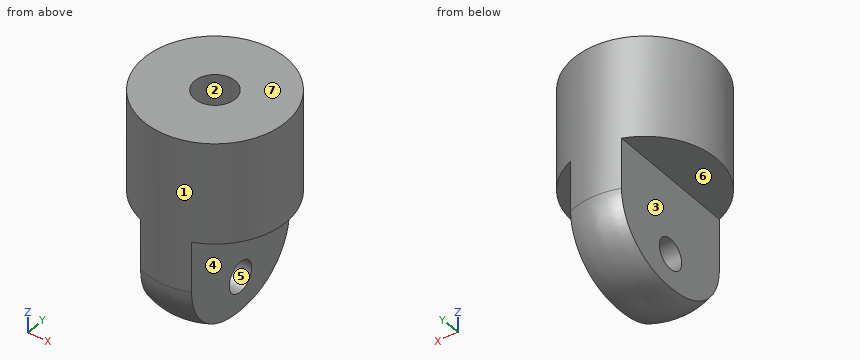
```python
from build123d import *

# Parameters (mm, degrees)
SKETCH2_R          = 4
CUT_EXTRUDE1_DEPTH = 30
SKETCH3_W          = 19.126095086
SKETCH3_H          = 32.253484506
SKETCH3_W_2        = 14.725893552
SKETCH3_H_2        = 25.816213186
CUT_EXTRUDE2_DEPTH = 15
SKETCH4_R          = 3
CUT_EXTRUDE3_DEPTH = 30


with BuildPart() as part:
    # Sketch1 → Revolve1 (revolve)
    with BuildSketch(Plane(origin=(0, 0, 0), x_dir=(0, 0, -1), z_dir=(1, 0, 0)), mode=Mode.PRIVATE) as revolve1_sk:
        with BuildLine():
            Line((0, 0), (0, 14))
            Line((0, 14), (30, 14))
            ThreePointArc((30, 14), (39.186081867, 9.751268794), (41.896907171, 0))
            Line((41.896907171, 0), (0, 0))
        make_face()
    revolve(revolve1_sk.sketch.rotate(Axis((0, 0, 8.753832377), (0, 0, -1)), 90), axis=Axis((0, 0, 8.753832377), (0, 0, -1)))

    # Sketch2 → Cut-Extrude1 (cut)
    with BuildSketch(Plane.XY):
        Circle(SKETCH2_R)
    extrude(amount=-CUT_EXTRUDE1_DEPTH, mode=Mode.SUBTRACT)

    # Sketch3 → Cut-Extrude2 (cut, symmetric)
    with BuildSketch(Plane(origin=(0, 0, 0), x_dir=(1, 0, 0), z_dir=(0, 1, 0))):
        with Locations((-14.563047543, 36.126742253)):
            Rectangle(SKETCH3_W, SKETCH3_H)
        with Locations((12.362946776, 32.908106593)):
            Rectangle(SKETCH3_W_2, SKETCH3_H_2)
    extrude(amount=CUT_EXTRUDE2_DEPTH, both=True, mode=Mode.SUBTRACT)

    # Sketch4 → Cut-Extrude3 (cut)
    with BuildSketch(Plane(origin=(5, 0, 0), x_dir=(0, 0, -1), z_dir=(1, 0, 0))):
        with Locations((35, 0)):
            Circle(SKETCH4_R)
    extrude(amount=-CUT_EXTRUDE3_DEPTH, mode=Mode.SUBTRACT)


solid = part.part
```
Geometry check sheet. Reference: the model listing, model coordinates, mm. Face numbers are marked on the shaded views. A direction names the side the tool comes from. Round coordinates to 2 decimals unless told otherwise and drop trailing zeros. Order: outer loops, then holes, each group sorted by start corner. A loop starts at its lowest first (then second) coordinate and runs counter-clockwise, first axis right, second up. Notation, with made-up numbers: M 26.5,59.25 L 35.5,59.25 A14 ccw 35.5,85.25 Z; hole C -5,57.5 d8. An arc over 180 degrees is marked long. Write item = value, one per line.
Q1. Depth check by flat-ended pin: pin 1 Ø7 at (x, y) = (-10, 1.5) entering from -Z; pin 2 Ø6.5 at (y, z) = (-5.5, -32.5) entering from +X; pin 3 Ø3.5 at (y, z) = (0, -35) entering from -X; pin 4 Ø6 at (x, y) = (-4.5, -8) entering from -Z. Enter the tip coordinate at first touch or a pass-through.
Answer block:
pin_1 = -20
pin_2 = 5
pin_3 = through
pin_4 = -41.29
Q2. Release check for a two-part mould opening along Z. For the marked faces 4, 5, 6 and 7 record: released by +Z, released by -Z, zero draft, split by the parting line, or undercut.
Answer block:
face_4 = zero draft
face_5 = undercut
face_6 = released by -Z
face_7 = released by +Z
Q3. Section check B-B (z = -3). Enter the section's corners in (x, y).
Answer block:
outline = C 0,0 d28; hole C 0,0 d8
Q4. Scan lines: line 1 (Y direction, x = 0, z = -16.5); line 2 (Z direction, x = -8.25, y = 5); line 3 (X direction, y = -1, z = -16). Record each from-to range of solid material in increasing order.
Answer block:
line_1 = -14 to -4, 4 to 14
line_2 = -20 to 0
line_3 = -13.96 to -3.87, 3.87 to 13.96
Q5. Section check D-D (x = -10.5). Enter the section's corners in (y, z), plus the area to 3 significant figures.
Answer block:
outline = M -9.26,-20 L 9.26,-20 L 9.26,0 L -9.26,0 Z
area = 370 mm^2
Q6. Section check C-C (x = -6.5). Enter the section's corners in (y, z).
Answer block:
outline = M -12.4,-20 L 12.4,-20 L 12.4,0 L -12.4,0 Z
Q7. Set-up check for the marked faces 1, 2 and 3: record each of +Z, -Z, +X, -X, +Y, -Y from which the full face is reachable in a straight line by a thin tool's end or side.
Answer block:
face_1 = +Z, -Z
face_2 = +Z
face_3 = -Z, -X, +Y, -Y
Q8. Section check A-A (z = -25.5). Enter the section's corners in (x, y), plus the area to 3 significant figures.
Answer block:
outline = M -5,-13.08 A14 ccw 5,-13.08 L 5,13.08 A14 ccw -5,13.08 Z; hole C 0,0 d8
area = 224 mm^2
